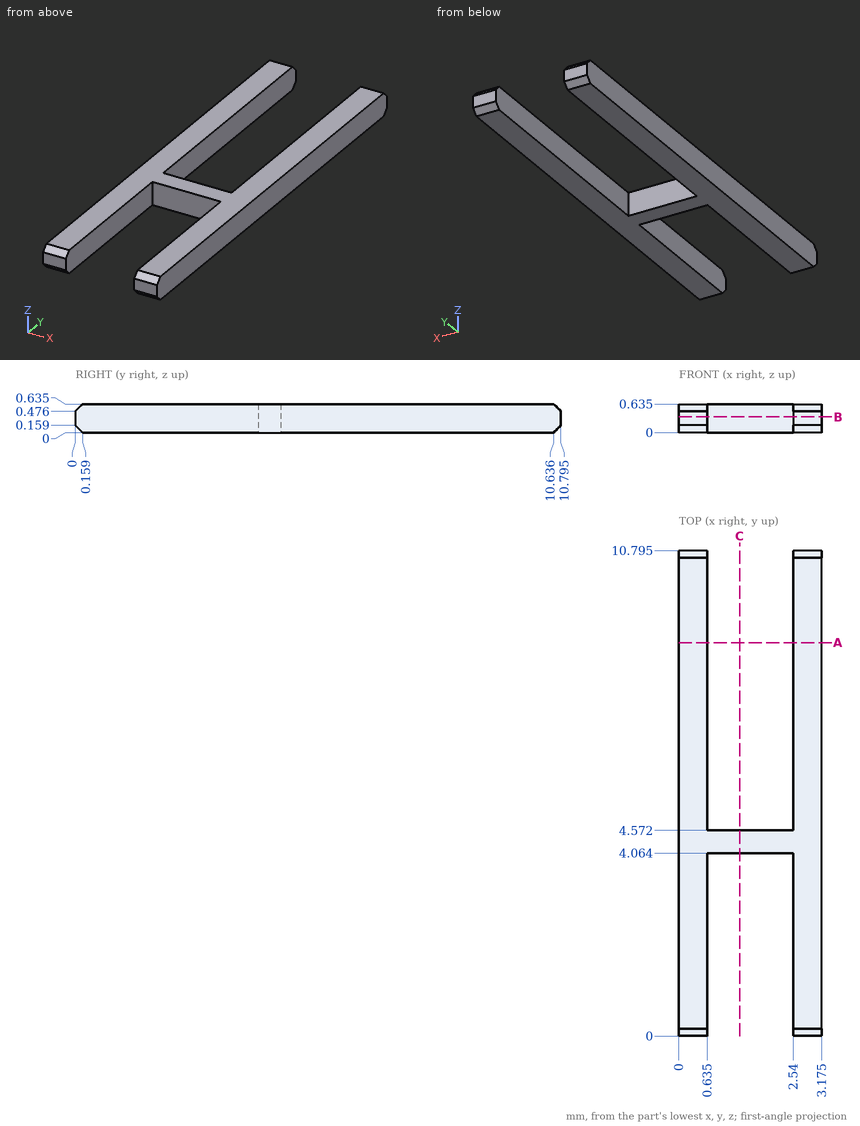
Print and shaded views of the part. All mm, measured from the part's lowest x, y and z. Coordinates: 2 decimals unless noted, no trailing zeros. Write each loop counter-clockwise with the first axis right and the second up, starting at its lowest first coordinate (ties: lowest second). Pieces come first, ordered by that corner, then holes. Notation, with made-up numbers: (74, -24) - (125, -24) arc R10 cw to (125, -8) - close; hole circle Ø11 at (-9, 11.25). An arc over 180 degrees is marked (long way). One line per question, with ' | ' between items. Start each with the question number.
Q1. Drill centre lines: line 1 (X direction, y = 9.5, z = 0.5) (1 decimal); line 2 (Y direction, x = 2.5, z = 0.35); line 3 (Y direction, x = 0.25, z = 0.5) (1 decimal). Where is each one in solid material? Low to high. Write a range as [from, to].
Q2. Cut at A-A, the plane y = 8.75. List the corners of the cut face in (x, z) (1 decimal).
Q3. Cut at B-B, the plane z = 0.35. List the corners of the cut face in (x, y) (1 decimal).
Q4. Cut at C-C, the plane x = 1.35. List the corners of the cut face in (y, z) (1 decimal).
Answer below:
1) line 1: [0, 0.6], [2.5, 3.2] | line 2: [4.06, 4.57] | line 3: [0, 10.8]
2) outline: (0, 0) - (0.6, 0) - (0.6, 0.6) - (0, 0.6) - close; (2.5, 0) - (3.2, 0) - (3.2, 0.6) - (2.5, 0.6) - close
3) outline: (0, 0) - (0.6, 0) - (0.6, 4.1) - (2.5, 4.1) - (2.5, 0) - (3.2, 0) - (3.2, 10.8) - (2.5, 10.8) - (2.5, 4.6) - (0.6, 4.6) - (0.6, 10.8) - (0, 10.8) - close
4) outline: (4.1, 0) - (4.6, 0) - (4.6, 0.6) - (4.1, 0.6) - close
